from build123d import *

# Parameters (mm, degrees)
SURFACE_EXTRUDE1_1_DEPTH = 120
THICKEN1_T2              = 15
SKETCH5_W                = 90
SKETCH5_H                = 120
CUT_EXTRUDE1_DEPTH       = 120
SKETCH4_W                = 120
SKETCH4_H                = 400
THICKEN2_T1              = 12
FILLET1_R                = 10
FILLET2_R                = 10
SKETCH6_R                = 5
BOSS_EXTRUDE1_DEPTH      = 40
CHAMFER1_SIZE            = 2
CHAMFER2_SIZE            = 2
SKETCH7_W                = 390
SKETCH7_H                = 120
BOSS_EXTRUDE2_DEPTH      = 40
CUT_EXTRUDE2_DEPTH       = 422
FILLET3_R                = 5
SKETCH9_W                = 3
SKETCH9_H                = 120
CUT_EXTRUDE3_DEPTH       = 440
FILLET4_R                = 2
FILLET5_R                = 2
FILLET6_R                = 2
SKETCH12_W               = 37
SKETCH12_H               = 120
CUT_EXTRUDE5_DEPTH       = 413
SKETCH13_W               = 30
SKETCH13_H               = 120
CUT_EXTRUDE6_DEPTH       = 20
SKETCH14_W               = 10
SKETCH14_H               = 120
BOSS_EXTRUDE3_DEPTH      = 7
FILLET7_R                = 10


with BuildPart() as body_1:
    # Surface-Extrude1: a surface, the sketch's curves swept straight by 120 mm
    with BuildLine(Plane(origin=(0, 0, 0), x_dir=(1, 0, 0), z_dir=(0, 1, 0)), mode=Mode.PRIVATE) as surface_extrude1_1_path:
        Line((60, -200), (-60, -200))
        Line((-60, -200), (-60, 200))
        Line((-60, 200), (60, 200))
        Line((60, 200), (60, -200))
    surface_extrude1_1 = Shell.extrude(surface_extrude1_1_path.wire(), (0 * SURFACE_EXTRUDE1_1_DEPTH, 1 * SURFACE_EXTRUDE1_1_DEPTH, 0 * SURFACE_EXTRUDE1_1_DEPTH))
    add(Solid.thicken(surface_extrude1_1, -THICKEN1_T2))

    # Sketch5 → Cut-Extrude1 (cut)
    with BuildSketch(Plane.XY.offset(-185)):
        with Locations((0, 60)):
            Rectangle(SKETCH5_W, SKETCH5_H)
    extrude(amount=-CUT_EXTRUDE1_DEPTH, mode=Mode.SUBTRACT)

    # Sketch4 → Surface-Plane1: a flat surface bounded by the sketch
    with BuildSketch(Plane(origin=(0, 0, 0), x_dir=(1, 0, 0), z_dir=(0, 1, 0)), mode=Mode.PRIVATE) as surface_plane1_2_region:
        Rectangle(SKETCH4_W, SKETCH4_H)
    surface_plane1_2 = surface_plane1_2_region.sketch.faces()[0]
    add(Solid.thicken(surface_plane1_2, THICKEN2_T1))

    # Fillet1
    fillet1_edges = [body_1.edges().sort_by_distance(p)[0] for p in [
        (45, 66, 185),
        (45, 12, -7.5),
        (-45, 66, 185),
        (0, 12, 185),
        (-45, 12, -7.5),
    ]]
    fillet(fillet1_edges, radius=FILLET1_R)

    # Fillet2
    fillet2_edges = [body_1.edges().sort_by_distance(p)[0] for p in [
        (60, 60, 200),
    ]]
    fillet(fillet2_edges, radius=FILLET2_R)

    # Sketch6 → Boss-Extrude1 (add)
    with BuildSketch(Plane(origin=(0, 0, -200), x_dir=(-1, 0, 0), z_dir=(0, 0, -1))):
        with Locations((-52.5, 100)):
            Circle(SKETCH6_R)
        with Locations((52.5, 100)):
            Circle(SKETCH6_R)
        with Locations((-52.5, 70)):
            Circle(SKETCH6_R)
        with Locations((-52.5, 40)):
            Circle(SKETCH6_R)
        with Locations((-52.5, 10)):
            Circle(SKETCH6_R)
        with Locations((52.5, 70)):
            Circle(SKETCH6_R)
        with Locations((52.5, 40)):
            Circle(SKETCH6_R)
        with Locations((52.5, 10)):
            Circle(SKETCH6_R)
    extrude(amount=BOSS_EXTRUDE1_DEPTH)

    # Chamfer1
    chamfer1_edges = [body_1.edges().sort_by_distance(p)[0] for p in [
        (57.5, 100, -240),
        (57.5, 70, -240),
        (57.5, 40, -240),
        (57.5, 10, -240),
    ]]
    chamfer(chamfer1_edges, length=CHAMFER1_SIZE)

    # Chamfer2
    chamfer2_edges = [body_1.edges().sort_by_distance(p)[0] for p in [
        (-47.5, 100, -240),
        (-47.5, 70, -240),
        (-47.5, 40, -240),
        (-47.5, 10, -240),
    ]]
    chamfer(chamfer2_edges, length=CHAMFER2_SIZE)

    # Sketch7 → Boss-Extrude2 (add)
    with BuildSketch(Plane(origin=(60, 0, 0), x_dir=(0, 0, -1), z_dir=(1, 0, 0))):
        with Locations((5, 60)):
            Rectangle(SKETCH7_W, SKETCH7_H)
    boss_extrude2 = extrude(amount=BOSS_EXTRUDE2_DEPTH)

    # Sketch8 → Cut-Extrude2 (cut)
    with BuildSketch(Plane(origin=(0, 0, -200), x_dir=(-1, 0, 0), z_dir=(0, 0, -1))):
        Polygon((-100, 105), (-100, 15), (-85, 15), (-90.773502692, 25), (-69.226497308, 25), (-75, 15), (-67, 15), (-67, 105), (-75, 105), (-69.226497308, 95), (-90.773502692, 95), (-85, 105), align=None)
    cut_extrude2 = extrude(amount=-CUT_EXTRUDE2_DEPTH, mode=Mode.SUBTRACT)

    # Fillet3
    fillet3_edges = [body_1.edges().sort_by_distance(p)[0] for p in [
        (60, 60, 190),
    ]]
    fillet(fillet3_edges, radius=FILLET3_R)

    # Sketch9 → Cut-Extrude3 (cut)
    with BuildSketch(Plane(origin=(0, 0, -200), x_dir=(-1, 0, 0), z_dir=(0, 0, -1))):
        with Locations((-98.5, 60)):
            Rectangle(SKETCH9_W, SKETCH9_H)
    cut_extrude3 = extrude(amount=-CUT_EXTRUDE3_DEPTH, mode=Mode.SUBTRACT)

    # Fillet4
    fillet4_edges = [body_1.edges().sort_by_distance(p)[0] for p in [
        (85, 105, -5),
        (75, 105, -5),
        (75, 15, -5),
        (85, 15, -5),
    ]]
    fillet(fillet4_edges, radius=FILLET4_R)

    # Fillet5
    fillet5_edges = [body_1.edges().sort_by_distance(p)[0] for p in [
        (69.226497308, 25, -5),
        (69.226497308, 95, -5),
    ]]
    fillet(fillet5_edges, radius=FILLET5_R)

    # Mirror1: Boss-Extrude2 across plane
    add(boss_extrude2.mirror(Plane(origin=(0, 0, 0), x_dir=(0, 0, 1), z_dir=(1, 0, 0))))

    # Mirror2: Cut-Extrude2 across plane
    add(cut_extrude2.mirror(Plane(origin=(0, 0, 0), x_dir=(0, 0, 1), z_dir=(1, 0, 0))), mode=Mode.SUBTRACT)

    # Fillet6
    fillet6_edges = [body_1.edges().sort_by_distance(p)[0] for p in [
        (-69.226497308, 25, -5),
        (-75, 15, -5),
        (-75, 105, -5),
        (-69.226497308, 95, -5),
        (-85, 105, -5),
        (-85, 15, -5),
    ]]
    fillet(fillet6_edges, radius=FILLET6_R)

    # Sketch12 → Cut-Extrude5 (cut)
    with BuildSketch(Plane(origin=(0, 0, -200), x_dir=(-1, 0, 0), z_dir=(0, 0, -1))):
        with Locations((-78.5, 60)):
            Rectangle(SKETCH12_W, SKETCH12_H)
    extrude(amount=-CUT_EXTRUDE5_DEPTH, mode=Mode.SUBTRACT)

    # Mirror3: Cut-Extrude3 across plane
    add(cut_extrude3.mirror(Plane(origin=(0, 0, 0), x_dir=(0, 0, 1), z_dir=(1, 0, 0))), mode=Mode.SUBTRACT)

    # Sketch13 → Cut-Extrude6 (cut)
    with BuildSketch(Plane.XY.offset(180)):
        with Locations((-82, 60)):
            Rectangle(SKETCH13_W, SKETCH13_H)
    extrude(amount=CUT_EXTRUDE6_DEPTH, mode=Mode.SUBTRACT)

    # Sketch14 → Boss-Extrude3 (add)
    with BuildSketch(Plane.ZY.offset(60)):
        with Locations((195, 60)):
            Rectangle(SKETCH14_W, SKETCH14_H)
    extrude(amount=BOSS_EXTRUDE3_DEPTH)

    # Fillet7
    fillet7_edges = [body_1.edges().sort_by_distance(p)[0] for p in [
        (-8.5, 0, 200),
        (55.773502692, 0, 198.164965809),
        (59.677903287, 0, 192.748194137),
    ]]
    fillet(fillet7_edges, radius=FILLET7_R)


solid = body_1.part
Build history of the part. All positions in model axes, mm. A direction names the side the tool comes from. Round coordinates to 2 decimals unless told otherwise and drop trailing zeros. Order: outer loops, then holes, each group sorted by start corner. A loop starts at its lowest first (then second) coordinate and runs counter-clockwise, first axis right, second up. Notation, with made-up numbers: M 78.25,87.25 L 109.25,87.25 A17 cw 109.25,94.25 Z; hole C -19,-30.75 d4. An arc over 180 degrees is marked long. Use CSV: the item, a comma, the result in double quotes. Start each with the question number.
(1) Mould opens along Y. For faces 1 (the face through (-47, 51, -200)), 2 (the face through (-0.49, 15.01, 182.15)), 3 (the face through (-9.32, 2.85, 196.99)) say: +Y half, -Y half, draft (parallel to the pull), parting line (faces both ways), or undercut.
(2) Drill centre lines: probe 1 along X at (y, z) = (56.5, 51.5); probe 2 along Y at (x, z) = (-82, 18); probe 3 along Y at (x, z) = (-73, -101.5). Where is each one in solid material? Low to high.
(3) Cut at D-D on y = 53. List the corners of the cut face in (x, z).
(4) Tool access for faces 4 (the face through (-82, 10, 180)), 5 (the face through (-51.849, 44.957, -218.734)), 6 (the face through (0, 70, 185)): list every direction of +Z, -Z, +X, -X, +Y, -Y with a clear straight run to the whole face (end or side of a thin tool).
(5) Flat gauge pins, fed straight in: P1, Ø20, axis at x = -87, y = 10, coming from the +Z side; P2, Ø21, axis at x = 17.5, z = 44, coming from the +Y side; P3, Ø12, axis at y = 58, z = -72.5, coming from the -X side. Where does each tip first touch, or does it go through?
(6) Cut at B-B on z = -17. List the corners of the cut face in (x, y).
(7) Cut at C-C on x = -10. List the corners of the cut face in (y, z), then the cut area to 3 significant figures.
(8) Cut at A-A on y = 110.5. List the corners of the cut face in (x, z).
Findings:
1,face 1,"undercut"
1,face 2,"+Y half"
1,face 3,"-Y half"
2,probe 1,"x = -67 to -45, 45 to 60"
2,probe 2,"y = 0 to 25, 95 to 120"
2,probe 3,"y = 0 to 15.64, 18.46 to 25, 95 to 101.54, 104.36 to 120"
3,outline,"M -67,-200 L -45,-200 L -45,175 A10 cw -35,185 L 35,185 A10 cw 45,175 L 45,-200 L 60,-200 L 60,192.2 A5 cw 59.43,193.33 A10 ccw 50,200 L -67,200 Z"
4,face 4,"+Z, -X, +Y, -Y"
4,face 5,"-Z"
4,face 6,"-Z, +Y"
5,P1,"stops at z = 180"
5,P2,"stops at y = 12"
5,P3,"stops at x = -67"
6,outline,"M -97,0 L 60,0 L 60,120 L 45,120 L 45,22 A10 cw 35,12 L -35,12 A10 cw -45,22 L -45,120 L -97,120 L -97,105 L -88.46,105 A2 cw -86.73,102 L -90.77,95 L -72.69,95 A2 ccw -70.96,98 L -73.27,102 A2 cw -71.54,105 L -67,105 L -67,15 L -71.54,15 A2 cw -73.27,18 L -70.96,22 A2 ccw -72.69,25 L -90.77,25 L -86.73,18 A2 cw -88.46,15 L -97,15 Z"
7,outline,"M 0,-200 L 12,-200 L 12,175 A10 cw 22,185 L 120,185 L 120,200 L 10,200 A10 ccw 0,190 Z"
7,area,"6,420 mm^2"
8,outline,"M -97,-200 L -45,-200 L -45,175 A10 cw -35,185 L 35,185 A10 cw 45,175 L 45,-200 L 60,-200 L 60,192.2 A5 cw 59.43,193.33 A10 ccw 50,200 L -67,200 L -67,180 L -97,180 Z"
